from build123d import *

# Parameters (mm, degrees)
SKETCH1_R                       = 1.6
BOSS_EXTRUDE1_DEPTH             = 4.3
FILLET1_R                       = 1
CUT_EXTRUDE1_DEPTH              = 2
BOSS_EXTRUDE2_DEPTH             = 4.3
SKETCH4_R                       = 8.4
CUT_EXTRUDE2_DEPTH              = 32.552755501
SKETCH5_W                       = 40
SKETCH5_H                       = 8
CUT_EXTRUDE3_DEPTH              = 32.552755501
MOVE_FACE1_DEPTH                = 4.3
BOSS_EXTRUDE3_START             = 4
BOSS_EXTRUDE3_DEPTH             = 4
SKETCH7_R                       = 2.15
CUT_EXTRUDE4_DEPTH              = 3.5
CUT_EXTRUDE5_DEPTH              = 3
SKETCH9_W                       = 21.650635094
SKETCH9_H                       = 3.5
CUT_EXTRUDE6_DEPTH              = 4
FILLET2_R                       = 1
CHAMFER1_SIZE                   = 0.5
CUT_EXTRUDE7_DEPTH              = 3.5
BOSS_EXTRUDE4_REACH             = 28.705
BOSS_EXTRUDE4_DIRECTION_2_DEPTH = 20
FILLET3_R                       = 3
FILLET4_R                       = 5
FILLET5_R                       = 0.5


# Read off the part's stored shape, not the designer's step: Move Face1
with BuildPart() as part:
    # Sketch1 → Boss-Extrude1 (new body)
    with BuildSketch(Plane(origin=(0, 0, 0), x_dir=(1, 0, 0), z_dir=(0, 1, 0))):
        with BuildLine():
            Line((0, 17.320508076), (-15, 8.660254038))
            Line((-15, 8.660254038), (-15, -8.660254038))
            Line((-15, -8.660254038), (-6.25, -13.712068893))
            Line((-6.25, -13.712068893), (-6.25, 0))
            ThreePointArc((-6.25, 0), (0, 6.25), (6.25, 0))
            Line((6.25, 0), (6.25, -13.712068893))
            Line((6.25, -13.712068893), (15, -8.660254038))
            Line((15, -8.660254038), (15, 8.660254038))
            Line((15, 8.660254038), (0, 17.320508076))
        make_face()
        with Locations(Location((0, 12.5, 0), (0, 0, 90))):
            Circle(SKETCH1_R, mode=Mode.SUBTRACT)
        with Locations(Location((10.825317547, 6.25, 0), (0, 0, 90))):
            Circle(SKETCH1_R, mode=Mode.SUBTRACT)
        with Locations(Location((10.825317547, -6.25, 0), (0, 0, 90))):
            Circle(SKETCH1_R, mode=Mode.SUBTRACT)
        with Locations(Location((-10.825317547, -6.25, 0), (0, 0, 90))):
            Circle(SKETCH1_R, mode=Mode.SUBTRACT)
        with Locations(Location((-10.825317547, 6.25, 0), (0, 0, 90))):
            Circle(SKETCH1_R, mode=Mode.SUBTRACT)
    extrude(amount=BOSS_EXTRUDE1_DEPTH)

    # Fillet1
    fillet1_edges = [part.edges().sort_by_distance(p)[0] for p in [
        (15, 2.15, -8.660254038),
        (15, 2.15, 8.660254038),
        (6.25, 2.15, 13.712068893),
        (-6.25, 2.15, 13.712068893),
        (-15, 2.15, 8.660254038),
        (-15, 2.15, -8.660254038),
        (0, 2.15, -17.320508076),
    ]]
    fillet(fillet1_edges, radius=FILLET1_R)

    # Sketch2 → Cut-Extrude1 (cut)
    with BuildSketch(Plane(origin=(0, 4.3, 0), x_dir=(1, 0, 0), z_dir=(0, 1, 0))):
        Polygon((0, 15.848631561), (-2.9, 14.174315781), (-2.9, 10.825684219), (0, 9.151368439), (2.9, 10.825684219), (2.9, 14.174315781), align=None)
        Polygon((13.725317547, 4.575684219), (13.725317547, 7.924315781), (10.825317547, 9.598631561), (7.925317547, 7.924315781), (7.925317547, 4.575684219), (10.825317547, 2.901368439), align=None)
        Polygon((13.725317547, -4.575684219), (10.825317547, -2.901368439), (7.925317547, -4.575684219), (7.925317547, -7.924315781), (10.825317547, -9.598631561), (13.725317547, -7.924315781), align=None)
        Polygon((-13.725317547, -4.575684219), (-13.725317547, -7.924315781), (-10.825317547, -9.598631561), (-7.925317547, -7.924315781), (-7.925317547, -4.575684219), (-10.825317547, -2.901368439), align=None)
        Polygon((-13.725317547, 7.924315781), (-13.725317547, 4.575684219), (-10.825317547, 2.901368439), (-7.925317547, 4.575684219), (-7.925317547, 7.924315781), (-10.825317547, 9.598631561), align=None)
    extrude(amount=-CUT_EXTRUDE1_DEPTH, mode=Mode.SUBTRACT)

    # Sketch3 → Boss-Extrude2 (add)
    with BuildSketch(Plane(origin=(0, 4.3, 0), x_dir=(1, 0, 0), z_dir=(0, 1, 0))):
        with BuildLine():
            Line((-15, -8.082903769), (-6.25, -11.980018086))
            Line((-6.25, -11.980018086), (6.25, -11.980018086))
            Line((6.25, -11.980018086), (15, -8.082903769))
            Line((15, -8.082903769), (20, -10.969655115))
            Line((20, -10.969655115), (20, -22.376680266))
            ThreePointArc((20, -22.376680266), (19.517914755, -23.540537003), (18.354058018, -24.022622248))
            Line((18.354058018, -24.022622248), (-18.354058018, -24.022622248))
            ThreePointArc((-18.354058018, -24.022622248), (-19.517914755, -23.540537003), (-20, -22.376680266))
            Line((-20, -22.376680266), (-20, -10.969655115))
            Line((-20, -10.969655115), (-15, -8.082903769))
        make_face()
    extrude(amount=-BOSS_EXTRUDE2_DEPTH)

    # Sketch4 → Cut-Extrude2 (cut, through all)
    with BuildSketch(Plane(origin=(0, 4.3, 0), x_dir=(1, 0, 0), z_dir=(0, 1, 0))):
        with Locations((0, -14.022622248)):
            Circle(SKETCH4_R)
    extrude(amount=-CUT_EXTRUDE2_DEPTH, mode=Mode.SUBTRACT)

    # Sketch5 → Cut-Extrude3 (cut, through all)
    with BuildSketch(Plane(origin=(0, 4.3, 0), x_dir=(1, 0, 0), z_dir=(0, 1, 0))):
        with Locations((0, -20.022622248)):
            Rectangle(SKETCH5_W, SKETCH5_H)
    extrude(amount=-CUT_EXTRUDE3_DEPTH, mode=Mode.SUBTRACT)

    # Move Face1 outline → Move Face1 (add)
    with BuildSketch(Plane(origin=(0, 0, 0), x_dir=(1, 0, 0), z_dir=(0, 1, 0))):
        Polygon((20, -10.969655115), (20, -5.196152423), (15, -2.309401077), (15, -8.082903769), align=None)
        Polygon((-15, -2.309401077), (-20, -5.196152423), (-20, -10.969655115), (-15, -8.082903769), align=None)
    extrude(amount=MOVE_FACE1_DEPTH)

    # Sketch6 → Boss-Extrude3 (add)
    with BuildSketch(Plane(origin=(0, 4.3, 0), x_dir=(1, 0, 0), z_dir=(0, 1, 0)).offset(BOSS_EXTRUDE3_START)):
        with BuildLine():
            Line((-20, -12.522622248), (-8.264986388, -12.522622248))
            ThreePointArc((-8.264986388, -12.522622248), (-8.396109903, -14.278236217), (-8.158431222, -16.022622248))
            Line((-8.158431222, -16.022622248), (-20, -16.022622248))
            Line((-20, -16.022622248), (-20, -12.522622248))
        make_face()
        with BuildLine():
            Line((8.264986388, -12.522622248), (20, -12.522622248))
            Line((20, -12.522622248), (20, -16.022622248))
            Line((20, -16.022622248), (8.158431222, -16.022622248))
            ThreePointArc((8.158431222, -16.022622248), (8.396109903, -14.278236217), (8.264986388, -12.522622248))
        make_face()
    extrude(amount=-BOSS_EXTRUDE3_DEPTH)

    # Sketch7 → Cut-Extrude4 (cut)
    with BuildSketch(Plane.XY.offset(16.022622248)):
        with Locations((-16, 3)):
            Circle(SKETCH7_R)
        with Locations((16, 3)):
            Circle(SKETCH7_R)
    extrude(amount=-CUT_EXTRUDE4_DEPTH, mode=Mode.SUBTRACT)

    # Sketch8 → Cut-Extrude5 (cut)
    with BuildSketch(Plane(origin=(0, 0, 12.522622248), x_dir=(-1, 0, 0), z_dir=(0, 0, -1))):
        Polygon((16, 6.290896534), (13.15, 4.645448267), (13.15, 1.354551733), (16, -0.290896534), (18.85, 1.354551733), (18.85, 4.645448267), align=None)
        Polygon((-18.85, 4.645448267), (-16, 6.290896534), (-13.15, 4.645448267), (-13.15, 1.354551733), (-16, -0.290896534), (-18.85, 1.354551733), align=None)
    extrude(amount=CUT_EXTRUDE5_DEPTH, mode=Mode.SUBTRACT)

    # Sketch9 → Cut-Extrude6 (cut)
    with BuildSketch(Plane(origin=(0, 4.3, 0), x_dir=(1, 0, 0), z_dir=(0, 1, 0))):
        with Locations((0, -14.272622248)):
            Rectangle(SKETCH9_W, SKETCH9_H)
    extrude(amount=CUT_EXTRUDE6_DEPTH, mode=Mode.SUBTRACT)

    # Fillet2
    fillet2_edges = [part.edges().sort_by_distance(p)[0] for p in [
        (20, 2.15, 5.196152423),
        (-20, 2.15, 5.196152423),
        (8.158431222, 2.15, 16.022622248),
        (20, 6.3, 12.522622248),
        (-20, 6.3, 12.522622248),
        (-8.158431222, 2.15, 16.022622248),
        (-10.825317547, 6.3, 16.022622248),
        (10.825317547, 6.3, 12.522622248),
        (-10.825317547, 6.3, 12.522622248),
        (10.825317547, 6.3, 16.022622248),
        (15, 2.15, 2.309401077),
        (-15, 2.15, 2.309401077),
    ]]
    fillet(fillet2_edges, radius=FILLET2_R)

    # Chamfer1
    chamfer1_edges = [part.edges().sort_by_distance(p)[0] for p in [
        (0, 4.3, -6.25),
        (6.25, 4.3, 4.205179445),
        (-6.25, 4.3, 4.205179445),
        (-6.25, 0, 4.205179445),
        (6.25, 0, 4.205179445),
        (0, 0, -6.25),
    ]]
    chamfer(chamfer1_edges, length=CHAMFER1_SIZE)

    # Sketch10 → Cut-Extrude7 (cut)
    with BuildSketch(Plane.XY.offset(16.022622248)):
        with BuildLine():
            Line((-17.52027958, 4.52027958), (-16, 6.040559159))
            Line((-16, 6.040559159), (-14.47972042, 4.52027958))
            ThreePointArc((-14.47972042, 4.52027958), (-16, 0.85), (-17.52027958, 4.52027958))
        make_face()
        with BuildLine():
            Line((14.47972042, 4.52027958), (16, 6.040559159))
            Line((16, 6.040559159), (17.52027958, 4.52027958))
            ThreePointArc((17.52027958, 4.52027958), (16, 0.85), (14.47972042, 4.52027958))
        make_face()
    extrude(amount=-CUT_EXTRUDE7_DEPTH, mode=Mode.SUBTRACT)

    # Boss-Extrude4: up to this face of the body (flat: up to its plane)
    boss_extrude4_end = Plane(part.part.faces().sort_by_distance((-8.607291251, 0, 11.682408659))[0])
    # Sketch11 → Boss-Extrude4 (add, up to the picked face)
    with BuildSketch(Plane(origin=(0, 4.3, 0), x_dir=(1, 0, 0), z_dir=(0, 1, 0)), mode=Mode.PRIVATE) as boss_extrude4_sk1:
        Polygon((9, -1.154700538), (19, -6.92820323), (19, -16.022622248), (21, -16.022622248), (21, -5.773502692), (9, 1.154700538), align=None)
    boss_extrude4_tool1 = split(extrude(boss_extrude4_sk1.sketch, amount=-BOSS_EXTRUDE4_REACH, mode=Mode.PRIVATE), bisect_by=boss_extrude4_end, keep=Keep.BOTH, mode=Mode.PRIVATE)
    # Sketch11 → Boss-Extrude4 (add, up to the picked face)
    with BuildSketch(Plane(origin=(0, 4.3, 0), x_dir=(1, 0, 0), z_dir=(0, 1, 0)), mode=Mode.PRIVATE) as boss_extrude4_sk2:
        Polygon((-9, 1.154700538), (-9, -1.154700538), (-19, -6.92820323), (-19, -16.022622248), (-21, -16.022622248), (-21, -5.773502692), align=None)
    boss_extrude4_tool2 = split(extrude(boss_extrude4_sk2.sketch, amount=-BOSS_EXTRUDE4_REACH, mode=Mode.PRIVATE), bisect_by=boss_extrude4_end, keep=Keep.BOTH, mode=Mode.PRIVATE)
    add(boss_extrude4_tool1.solids().sort_by(Axis((14.104769, 4.3, 3.859987), (0, -1, 0)))[0])
    add(boss_extrude4_tool2.solids().sort_by(Axis((-9.209538, 4.3, 0), (0, -1, 0)))[0])

    # Sketch11 → Boss-Extrude4 direction 2 (add)
    with BuildSketch(Plane(origin=(0, 4.3, 0), x_dir=(1, 0, 0), z_dir=(0, 1, 0))):
        Polygon((9, -1.154700538), (19, -6.92820323), (19, -16.022622248), (21, -16.022622248), (21, -5.773502692), (9, 1.154700538), align=None)
        Polygon((-9, 1.154700538), (-9, -1.154700538), (-19, -6.92820323), (-19, -16.022622248), (-21, -16.022622248), (-21, -5.773502692), align=None)
    extrude(amount=BOSS_EXTRUDE4_DIRECTION_2_DEPTH)

    # Fillet3
    fillet3_edges = [part.edges().sort_by_distance(p)[0] for p in [
        (19, 14.3, 6.92820323),
        (-19, 14.3, 6.92820323),
    ]]
    fillet(fillet3_edges, radius=FILLET3_R)

    # Fillet4
    fillet4_edges = [part.edges().sort_by_distance(p)[0] for p in [
        (21, 12.15, 5.773502692),
        (-21, 12.15, 5.773502692),
    ]]
    fillet(fillet4_edges, radius=FILLET4_R)

    # Fillet5
    fillet5_edges = [part.edges().sort_by_distance(p)[0] for p in [
        (9, 14.3, -1.154700538),
        (9, 14.3, 1.154700538),
        (19, 16.3, 16.022622248),
        (21, 12.15, 16.022622248),
        (-9, 14.3, -1.154700538),
        (-21, 12.15, 16.022622248),
        (-19, 16.3, 16.022622248),
        (-9, 14.3, 1.154700538),
    ]]
    fillet(fillet5_edges, radius=FILLET5_R)


solid = part.part
For this review, take the finished solid that the model builds, in its own axes (mm). A direction names the side the tool comes from. Give positions to 0.01 mm unless a question says otherwise; leave off trailing zeros. Order: outer loops, then holes, each group sorted by start corner. A loop starts at its lowest first (then second) coordinate and runs counter-clockwise, first axis right, second up. Notation, with made-up numbers: (20, -6) -> (38, -6) arc R20 cw to (38, 12) -> close; hole circle Ø7 at (-32.5, 44). An arc over 180 degrees is marked (long way). Write item = value, one per line.
1) We need section B-B, the plane z = -5.5. Count the separate pieces of the cut face and the enclosed holes in it, and give its area (3 significant figures).
Findings:
separate_pieces = 4
enclosed_holes = 0
area = 66.3 mm^2
2) Draft analysis for pull direction X (two halves, no side actions). For faces 4 (the face through (7.598, 2.12, -12.934)), 5 (the face through (12.245, 1.134, 5.512)), state which applies: pulls with the +X half, pulls with the -X half, needs draft (parallel to the pull), parting line crosses it, or undercut.
Findings:
face_4 = pulls with the +X half
face_5 = undercut
3) Insertion check: pin 1 (1 mm diameter, centred on x = -16, y = 16, fed in from -Z); pin 2 (8 mm diameter, centred on x = -6.5, z = -2, fed in from +Y); pin 3 (2 mm diameter, centred on y = 3, z = -9.5, fed in from -X); pin 4 (3 mm diameter, centred on x = 9.5, z = -7.5, fed in from +Y). Each pin has a flat end and moves straight along its axis. Give the tip position at first contact, or say it passes through.
Findings:
pin_1 = 2.6
pin_2 = 24.3
pin_3 = -14.91
pin_4 = 4.3
4) For faces 1 (the face through (-6.25, 2, 4)), 2 (the face through (-16.77, 5.27, 14.3)), 3 (the face through (-11.126, 6.328, 12.808)), list the 3-axis set-ups (+Z, -Z, +X, -X, +Y, -Y) from which the entire face can be reached by the end or side of a thin tool; tool diameter is ignored.
Findings:
face_1 = +Z, +Y, -Y
face_2 = +Z
face_3 = +Y
5) To check wall thickness, follow L1, parallel to X at y = 13.5, z = 12; L2, parallel to X at y = 3.75, z = -7.5; L3, parallel to X at y = 1.85, z = 6.25. State the ranges of each line that lie inside material, in increasing order. Write a range as from..to.
Findings:
L1 = -21..-19, 19..21
L2 = -15..-13.73, -7.93..7.93, 13.73..15
L3 = -20.38..-12.43, -9.23..-6.25, 6.25..9.23, 12.43..20.38
6) We need section A-A, the plane x = 17. Give the boundary of the cut face in (y, z).
Findings:
outline = (0, 3.46) -> (24.3, 3.46) -> (24.3, 5.77) -> (4.3, 5.77) -> (4.3, 9.52) -> (0.29, 9.52) -> (0.29, 12.52) -> (1.1, 12.52) -> (1.1, 16.02) -> (0, 16.02) -> close; (5.04, 12.52) -> (8.3, 12.52) -> (8.3, 16.02) -> (5.04, 16.02) -> close
